Geometry check sheet. Reference: the model listing, model coordinates, mm. Coordinates: 2 decimals unless noted, no trailing zeros. Loops run counter-clockwise (first coordinate to the right, second up) from the corner with the lowest first, then second, coordinate; pieces in that order, holes last.
Autodesk Inventor part; units mm, degrees
ref_plane "YZ Plane" through (0, 0, 0) normal (1, 0, 0) x (0, 1, 0)
ref_plane "XZ Plane" through (0, 0, 0) normal (0, 1, 0) x (-1, 0, 0)
ref_plane "XY Plane" through (0, 0, 0) normal (0, 0, 1) x (1, 0, 0)
sketch "Sketch1" plane through (0, 0, 0) normal (1, 0, 0) x (0, 1, 0)
  line L0 (2812.3869, 0) -> (2812.3869, -5171.1623) construction
  line L1 (2812.3869, -5171.1623) -> (0, -5171.1623) construction
  line L2 (0, -5171.1623) -> (0, 0) construction
  line L3 (0, 0) -> (2812.3869, 0) construction
  point P0 (0, 0)
sketch "Sketch3" plane through (0, 0, 0) normal (1, 0, 0) x (0, 1, 0)
  arc A0 (670.9217, -1192.002) -> (490.3182, -1294.4333) centre (735.6427, -1516.5486) ccw
  circle A1 centre (699.299, -1221.9874) radius 15
  circle A2 centre (485.0015, -1332.1305) radius 15
  line L0 (670.9217, -1192.002) -> (694.5217, -1189.6422)
  line L1 (694.5217, -1189.6422) -> (719.5378, -1192.8832)
  line L2 (719.5378, -1192.8832) -> (733.6455, -1211.4411)
  line L3 (733.6455, -1211.4411) -> (735.5916, -1230.9034)
  line L4 (735.5916, -1230.9034) -> (721.8585, -1246.2211)
  line L5 (721.8585, -1246.2211) -> (706.6308, -1251.2582)
  line L6 (706.6308, -1251.2582) -> (677.2013, -1248.7397)
  line L7 (677.2013, -1248.7397) -> (657.762, -1246.2211)
  line L8 (657.762, -1246.2211) -> (534.9682, -1320.4431)
  line L9 (534.9682, -1320.4431) -> (521.9986, -1334.9093)
  line L10 (521.9986, -1334.9093) -> (513.5108, -1351.8536)
  line L11 (513.5108, -1351.8536) -> (502.7761, -1360.014)
  line L12 (502.7761, -1360.014) -> (482.1715, -1362.0744)
  line L13 (482.1715, -1362.0744) -> (466.9183, -1354.4337)
  line L14 (466.9183, -1354.4337) -> (460.8027, -1339.4632)
  line L15 (460.8027, -1339.4632) -> (463.2669, -1320.4431)
  line L16 (463.2669, -1320.4431) -> (474.5449, -1307.8638)
  line L17 (474.5449, -1307.8638) -> (486.2652, -1298.954)
  line L18 (486.2652, -1298.954) -> (490.3182, -1294.4333)
  point P0 (0, 0)
  dimension "d9" = 30
  dimension "d10" = 30
extrude "Extrusion2" add sketch "Sketch3" along normal mid plane 150
fillet "Fillet1" radius 20 2 edges at (0, 657.762, -1246.2211) (0, 534.9682, -1320.4431)
fillet "Fillet2" radius 2 42 edges at (75, 572.3788, -1228.6872) (75, 488.2917, -1296.6937) (75, 480.405, -1303.4089) (75, 468.9059, -1314.1535) (75, 462.0348, -1329.9531) (75, 463.8605, -1346.9484) (75, 474.5449, -1358.254) (75, 492.4738, -1361.0442) (75, 508.1435, -1355.9338) (75, 517.7547, -1343.3815) (75, 527.4874, -1328.7871) (75, 535.1095, -1320.6136) (75, 594.6506, -1284.3684) (75, 670.948, -1247.9295) (75, 691.916, -1249.9989) (75, 714.2446, -1248.7397) (75, 728.725, -1238.5623) (75, 734.6185, -1221.1723) (75, 726.5916, -1202.1622) (75, 707.0298, -1191.2627) (75, 682.7217, -1190.8221) (-75, 572.3788, -1228.6872) (-75, 682.7217, -1190.8221) (-75, 707.0298, -1191.2627) (-75, 726.5916, -1202.1622) (-75, 734.6185, -1221.1723) (-75, 728.725, -1238.5623) (-75, 714.2446, -1248.7397) (-75, 691.916, -1249.9989) (-75, 670.948, -1247.9295) (-75, 594.6506, -1284.3684) (-75, 535.1095, -1320.6136) (-75, 527.4874, -1328.7871) (-75, 517.7547, -1343.3815) (-75, 508.1435, -1355.9338) (-75, 492.4738, -1361.0442) (-75, 474.5449, -1358.254) (-75, 463.8605, -1346.9484) (-75, 462.0348, -1329.9531) (-75, 468.9059, -1314.1535) (-75, 480.405, -1303.4089) (-75, 488.2917, -1296.6937)
fillet "Fillet3" radius 2 6 edges at (0, 719.5378, -1192.8832) (0, 733.6455, -1211.4411) (74.4142, 719.2197, -1193.4327) (-74.4142, 719.2197, -1193.4327) (74.4142, 733.079, -1211.6639) (-74.4142, 733.079, -1211.6639)
properties part number "Lankarm_lång"
1) Depth check by flat-ended pin: pin 1 (1.5 mm diameter, centred on x = -18, y = 575, fed in from +Z); pin 2 (12 mm diameter, centred on y = 564.5, z = -1313.5, fed in from -X); pin 3 (12 mm diameter, centred on x = 56.5, z = -1328.5, fed in from -Y); pin 4 (4 mm diameter, centred on x = -29.5, z = -1285, fed in from +Y). Enter the tip coordinate at first touch or a pass-through.
Data:
pin 1: stops at z = -1226.8
pin 2: passes through
pin 3: stops at y = 461.45
pin 4: stops at y = 596.91
2) Material ranges on probe 1 along Y at (x, z) = (1.5, -1327); probe 2 along Y at (x, z) = (-43, -1336); probe 3 along Z at (x, y) = (32, 689.5), recorded low to high.
Data:
probe 1: y = 462.42 to 470.91, 499.1 to 529.09
probe 2: y = 461.25 to 470.51, 499.49 to 521.45
probe 3: z = -1249.79 to -1233.34, -1210.63 to -1190.14
3) Mould release check, pull along Z, two halves, no side actions. Record for faces 1 (the cylindrical face through (-1.05, 696.047, -1207.344)), 2 (the flat face through (-75, 588, -1263)), 3 (the flat face through (-1.02, 682.56, -1190.84)): +Z half, -Z half, draft (parallel to the pull), parting line (faces both ways), or undercut.
Data:
face 1: undercut
face 2: draft
face 3: +Z half
4) Section check A-A on x = -38.5. Record the cut outline in (y, z), and give its area (3 significant figures).
Data:
outline: (460.8, -1339.46) - (466.92, -1354.43) - (482.17, -1362.07) - (502.78, -1360.01) - (513.51, -1351.85) - (522, -1334.91) - (532.98, -1322.66) arc R20 cw to (537.52, -1318.9) - (651.78, -1249.84) arc R20 cw to (664.69, -1247.12) - (677.2, -1248.74) - (706.63, -1251.26) - (721.86, -1246.22) - (735.59, -1230.9) - (733.7, -1212) arc R2 ccw to (733.3, -1210.99) - (720.04, -1193.55) arc R2 ccw to (718.71, -1192.78) - (694.52, -1189.64) - (670.92, -1192) arc R330.94 ccw to (490.32, -1294.43) - (486.27, -1298.95) - (474.54, -1307.86) - (463.27, -1320.44) - close; hole circle Ø30 at (485, -1332.13); hole circle Ø30 at (699.3, -1221.99)
area: 15,300 mm2
